The figure shows three views and two pictorial views of one solid part (mm, origin at its lowest corner). Answer the questions. Coordinates: 2 decimals unless noted, no trailing zeros. Write each loop counter-clockwise with the first axis right and the second up, starting at its lowest first coordinate (ties: lowest second). Pieces come first, ordered by that corner, then holes. Notation, with made-up numbers: M 55.5,69.25 L 76.5,69.25 A17 cw 76.5,73.25 Z; hole C -25,31 d1. An arc over 180 degrees is marked long. Use CSV: the item, a comma, the result in double quotes.
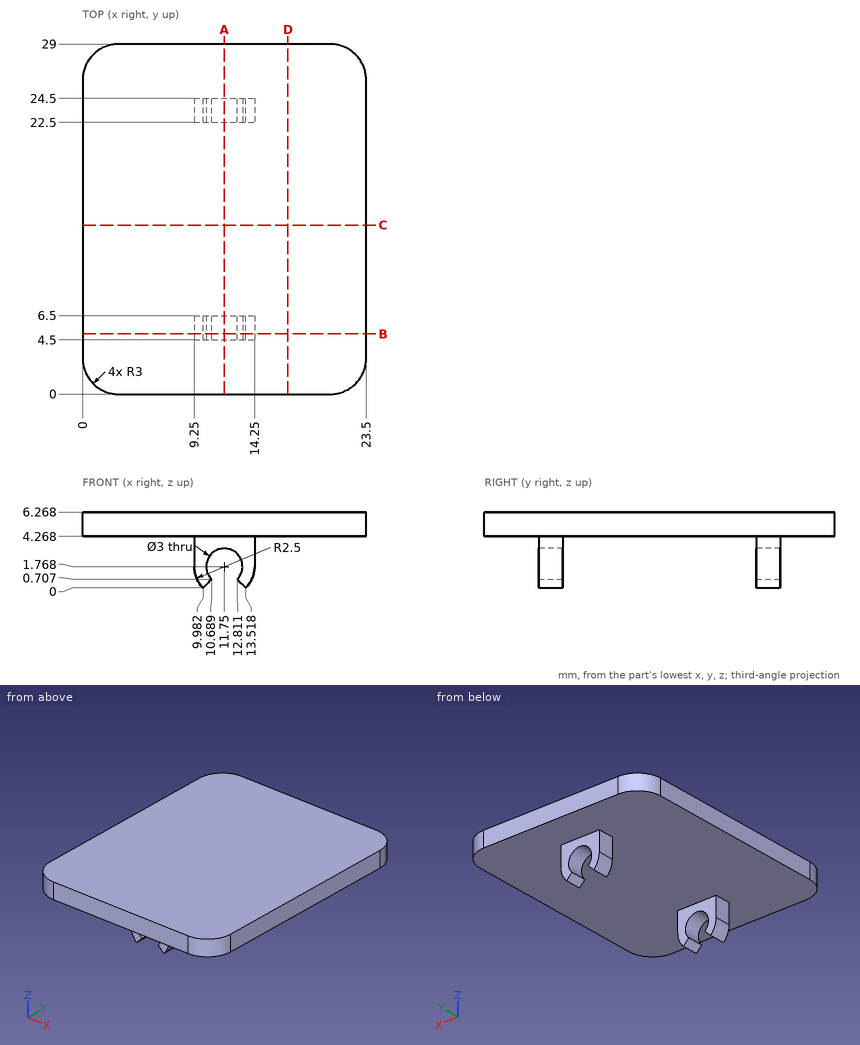
Item 1: The part is cut by section A-A (x = 11.75). Write down the section's boundary in (y, z), then the cut area to 3 significant figures.
Answer:
outline,"M 0,4.27 L 4.5,4.27 L 4.5,3.27 L 6.5,3.27 L 6.5,4.27 L 22.5,4.27 L 22.5,3.27 L 24.5,3.27 L 24.5,4.27 L 29,4.27 L 29,6.27 L 0,6.27 Z"
area,"62.0 mm2"
Item 2: Consider probe 1 along Y at (x, z) = (9.5, 1); probe 2 along Z at (x, y) = (9.5, 2.25); probe 3 along Z at (x, y) = (11.75, 5.7). Determine where each line is inside the solid, lowest interval first.
Answer:
probe 1,"y = 4.5 to 6.5, 22.5 to 24.5"
probe 2,"z = 4.27 to 6.27"
probe 3,"z = 3.27 to 6.27"
Item 3: The part is cut by section D-D (x = 17). Write down the section's boundary in (y, z).
Answer:
outline,"M 0,4.27 L 29,4.27 L 29,6.27 L 0,6.27 Z"
Item 4: The part is cut by section B-B (y = 5). Write down the section's boundary in (x, z).
Answer:
outline,"M 0,4.27 L 9.25,4.27 L 9.25,1.77 A2.5 ccw 9.98,0 L 10.69,0.71 A1.5 cw long 12.81,0.71 L 13.52,0 A2.5 ccw 14.25,1.77 L 14.25,4.27 L 23.5,4.27 L 23.5,6.27 L 0,6.27 Z"
Item 5: Given pin 1 (0.6 mm diameter, centred on y = 23.5, z = 3, fed in from +X); pin 2 (1 mm diameter, centred on y = 5.5, z = 2.5, fed in from -X); pin 3 (1.8 mm diameter, centred on x = 11.75, z = 1.77, fed in from -Y); pin 4 (2 mm diameter, centred on x = 11, z = 2.5, fed in from +Y), each flat-ended and moving along its own axis, determine where each tip first touches the part or whether it passes through.
Answer:
pin 1,"stops at x = 14.25"
pin 2,"stops at x = 9.25"
pin 3,"passes through"
pin 4,"stops at y = 24.5"
Item 6: The part is cut by section C-C (y = 14). Write down the section's boundary in (x, z), then the cut area to 3 significant figures.
Answer:
outline,"M 0,4.27 L 23.5,4.27 L 23.5,6.27 L 0,6.27 Z"
area,"47.0 mm2"
